```python
from build123d import *

# Parameters (mm, degrees)
BOSS_EXTRUDE1_START = -10
BOSS_EXTRUDE1_DEPTH = 20


# Read off the part's stored shape, not the designer's step: Boss-Extrude1
with BuildPart() as part:
    # Boss-Extrude1 outline → Boss-Extrude1 (new body)
    with BuildSketch(Plane(origin=(0, 0, 0), x_dir=(1, 0, 0), z_dir=(0, 1, 0)).offset(BOSS_EXTRUDE1_START)):
        with BuildLine():
            Line((-12.534244987, 10), (0, 10))
            Line((0, 10), (0, 20))
            Line((0, 20), (-30, 20))
            Line((-30, 20), (-35, 15))
            Line((-35, 15), (-35, 7.5))
            Line((-35, 7.5), (-32.803300859, 5.303300859))
            ThreePointArc((-32.803300859, 5.303300859), (-24.629874257, 6.929096494), (-20, 0))
            Line((-20, 0), (-18.307747679, 0))
            Line((-18.307747679, 0), (-12.534244987, 10))
        make_face()
    extrude(amount=BOSS_EXTRUDE1_DEPTH)

    # Mirror2: part across plane


with BuildPart() as part_1:
    add(part.part)
    add(part.part.mirror(Plane(origin=(0, 0, 0), x_dir=(0, 0, 1), z_dir=(1, 0, 0))))


solid = part_1.part
```
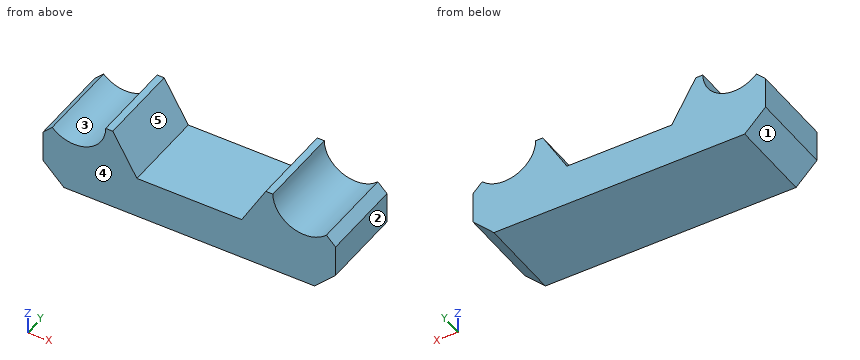
Input: part model. Units: mm. Frame: model coordinates. Face numbers are marked on the shaded views. A direction names the side the tool comes from. Give positions to 0.01 mm unless a question says otherwise; leave off trailing zeros. Loops run counter-clockwise (first coordinate to the right, second up) from the corner with the lowest first, then second, coordinate; pieces in that order, holes last. Notation, with made-up numbers: M 28,52 L 35,52 A21 ccw 35,67 Z; hole C 48,-22.5 d6. An arc over 180 degrees is marked long. Answer as CSV lines item,"result". Start each with the question number.
1. Section A-A on z = -6.75. Return loops of the section in (x, y), plus the area to 3 significant figures.
2. Section D-D on x = -7.5. Return loops of the section in (y, z).
3. Section B-B on y = -7.5. Return loops of the section in (x, z), plus the area to 3 significant figures.
4. Line query: L1, parallel to X at y = 5, z = -5.5; L2, parallel to X at y = -4.5, z = -6.5; L3, parallel to Z at x = 1.5, y = 5.5. Output: solid intervals per line, ascending.
5. Reachability of the marked faces 4 and 5 from +Z, -Z, +X, -X, +Y, -Y: full face, straight path, thin tool, end or side. Return the list, or none.
6. Section C-C on z = -16.5. Return loops of the section in (x, y).
7. Pull-direction query (X, two-part tool) for the marked faces 1, 2 and 3; classes: released by +X, released by -X, zero draft, split by the parting line, or undercut.
8. Pin query (flat end, axial travel): P1, Ø6, axis at x = -6.5, z = -4.5, coming from the -Y side; P2, Ø6, axis at x = 1, y = 4.5, coming from the +Z side. Return the tip coordinate at first contact, or that it passes through.
Computed values:
1,outline,"M -34.25,-10 L -30.77,-10 L -30.77,10 L -34.25,10 Z; M -24.23,-10 L -14.41,-10 L -14.41,10 L -24.23,10 Z; M 14.41,-10 L 24.23,-10 L 24.23,10 L 14.41,10 Z; M 30.77,-10 L 34.25,-10 L 34.25,10 L 30.77,10 Z"
1,area,"532 mm²"
2,outline,"M -10,-20 L 10,-20 L 10,-10 L -10,-10 Z"
3,outline,"M -35,-15 L -30,-20 L 30,-20 L 35,-15 L 35,-7.5 L 32.8,-5.3 A7.5 cw 20,0 L 18.31,0 L 12.53,-10 L -12.53,-10 L -18.31,0 L -20,0 A7.5 cw -32.8,-5.3 L -35,-7.5 Z"
3,area,"878 mm²"
4,L1,"x = -33 to -32.6, -22.4 to -15.13, 15.13 to 22.4, 32.6 to 33"
4,L2,"x = -34 to -31.24, -23.76 to -14.55, 14.55 to 23.76, 31.24 to 34"
4,L3,"z = -20 to -10"
5,face 4,"+Z, -Z, +X, -X, -Y"
5,face 5,"+Z, +Y, -Y"
6,outline,"M -33.5,-10 L 33.5,-10 L 33.5,10 L -33.5,10 Z"
7,face 1,"released by -X"
7,face 2,"released by +X"
7,face 3,"undercut"
8,P1,"passes through"
8,P2,"stops at z = -10"
